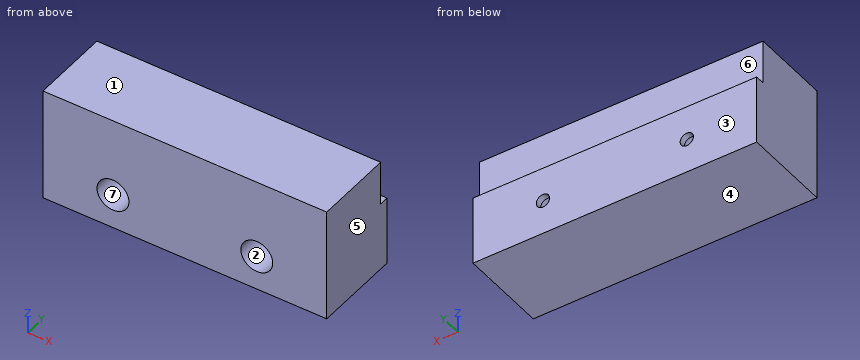
```python
from build123d import *

# Parameters (mm, degrees)
F1_DEPTH = 101.6
F2_R     = 2.38125
F3_DEPTH = 6.35
F4_R     = 5.715
F5_DEPTH = 4.064
F6_DEPTH = 25.4
F7_DEPTH = 23.7960387021


with BuildPart() as f1:
    # F0 (on Right) → F1 (new body)
    with BuildSketch(Plane.YZ):
        Polygon((0, -31.1910395777), (0, -15.3160395777), (-2.9972, -15.3160395777), (-2.9972, -55.9560395777), (3.3528, -55.9560395777), (3.3528, -31.1910395777), align=None)
    extrude(amount=F1_DEPTH)

    # F2 (on face) → F3 (cut, through all)
    with BuildSketch(Plane(origin=(0, 3.3528, 0), x_dir=(-1, 0, 0), z_dir=(0, 1, 0))):
        with Locations((-76.5522494912, -43.5735395777)):
            Circle(F2_R)
        with Locations((-25.0477505088, -43.5735395777)):
            Circle(F2_R)
    extrude(amount=-F3_DEPTH, mode=Mode.SUBTRACT)

    # F4 (on face) → F5 (cut)
    with BuildSketch(Plane.XZ.offset(2.9972)):
        with Locations((25.0477505088, -43.5735395777)):
            Circle(F4_R)
        with Locations((76.5522494912, -43.5735395777)):
            Circle(F4_R)
    extrude(amount=-F5_DEPTH, mode=Mode.SUBTRACT)

    # F6 (add): a face of the model
    f6_faces = [f1.faces().sort_by_distance(p)[0] for p in [
        (50.8, -2.9972, -35.2209054991),
    ]]
    extrude(f6_faces, amount=F6_DEPTH)

    # F7 (cut): a face of the model
    f7_faces = [f1.faces().sort_by_distance(p)[0] for p in [
        (50.8, -14.1986, -15.3160395777),
    ]]
    extrude(f7_faces, amount=F7_DEPTH, mode=Mode.SUBTRACT)


solid = f1.part
```
Work out the finished part from the listing and answer in its coordinate system (mm). Face numbers are marked on the shaded views. A direction names the side the tool comes from. Round coordinates to 2 decimals unless told otherwise and drop trailing zeros. Write each loop counter-clockwise with the first axis right and the second up, starting at its lowest first coordinate (ties: lowest second). Pieces come first, ordered by that corner, then holes. Notation, with made-up numbers: (57, 33) -> (115, 33) arc R8 cw to (115, 42) -> close; hole circle Ø7 at (-17, 0). An arc over 180 degrees is marked (long way). Write each question's results on one line, items separated by ' | '.
Q1. Section A-A, the plane x = 65 is taken. Write down the section's boundary in (y, z), then the cut area to 3 significant figures.
Data:
outline: (-28.4, -55.96) -> (3.35, -55.96) -> (3.35, -31.19) -> (0, -31.19) -> (0, -15.32) -> (-28.4, -15.32) -> close | area: 1,240 mm^2
Q2. Section B-B, the plane y = -20.5 is taken. Write down the section's boundary in (x, z) (3 decimals), then the cut area to 3 significant figures.
Data:
outline: (0, -55.956) -> (101.6, -55.956) -> (101.6, -15.316) -> (0, -15.316) -> close; hole circle Ø11.43 at (25.048, -43.574); hole circle Ø11.43 at (76.552, -43.574) | area: 3,920 mm^2
Q3. Straight lines are drawn through the part: line 1 along X through (y, z) = (1.5, -43.5); line 2 along Z through (x, y) = (76.5, -3.5); line 3 along X through (y, z) = (-20, -40.5). For each, find the intervals that lie inside material, in ascending order. Write a range as [from, to].
Data:
line 1: [0, 22.67], [27.43, 74.17], [78.93, 101.6] | line 2: [-55.96, -49.29], [-37.86, -15.32] | line 3: [0, 20.23], [29.87, 71.73], [81.37, 101.6]
Q4. Which of the six approach directions +Z, -Z, +X, -X, +Y, -Y give full straight-line access (tool end or side, diameter ignored) to the marked faces 5, 6 and 7?
Data:
face 5: +Z, -Z, +X, +Y, -Y | face 6: +Z, +X, -X, +Y | face 7: -Y
Q5. Section C-C, the plane z = -29 is taken. Write down the section's boundary in (x, y).
Data:
outline: (0, -28.4) -> (101.6, -28.4) -> (101.6, 0) -> (0, 0) -> close
Q6. A flat-ended cylindrical pin translates along its axis: P1, Ø6, axis at x = 25.05, z = -43.57, coming from the -Y side. Find the tip coordinate at first contact, or state that the pin passes through.
Data:
P1: y = 1.07
Q7. Determine the mould class of the marked faces 1, 2, 3 and 4 for opening direction Z: released by +Z, released by -Z, zero draft, split by the parting line, or undercut.
Data:
face 1: released by +Z | face 2: undercut | face 3: zero draft | face 4: released by -Z
